Here's how the part is built. I have some questions about the finished solid (model axes, mm). A direction names the side the tool comes from. Coordinates: 2 decimals unless noted, no trailing zeros. Write each loop counter-clockwise with the first axis right and the second up, starting at its lowest first coordinate (ties: lowest second). Pieces come first, ordered by that corner, then holes. Notation, with made-up numbers: M -30,24.5 L -15,24.5 A12 cw -15,40.5 Z; hole C 81.5,87 d10. An arc over 180 degrees is marked long. Use a Markdown table: item, result.
```python
from build123d import *

# Parameters (mm, degrees)
ESQUISSE1_R             = 110
BOSS_EXTRU_1_DEPTH      = 50
BOSS_EXTRU_2_DEPTH      = 50
ESQUISSE3_R             = 20
ENL_V_MAT_EXTRU_1_DEPTH = 456.460206824
BOSS_EXTRU_3_DEPTH      = 30
BOSS_EXTRU_4_DEPTH      = 85


with BuildPart() as part:
    # Esquisse1 → Boss.-Extru.1 (new body)
    with BuildSketch(Plane(origin=(0, 0, 0), x_dir=(1, 0, 0), z_dir=(0, 1, 0))):
        with Locations(Location((0, 0, 0), (0, 0, 270))):
            Circle(ESQUISSE1_R)
    extrude(amount=BOSS_EXTRU_1_DEPTH)

    # Esquisse2 → Boss.-Extru.2 (add, symmetric)
    with BuildSketch(Plane.XY):
        with BuildLine():
            Line((-70, 45), (70, 45))
            Line((70, 45), (60, 352))
            ThreePointArc((60, 352), (0, 412), (-60, 352))
            Line((-60, 352), (-70, 45))
        make_face()
    extrude(amount=BOSS_EXTRU_2_DEPTH, both=True)

    # Esquisse3 → Enl_v. mat.-Extru.1 (cut, through all)
    with BuildSketch(Plane.XY.offset(50)):
        with Locations((0, 352)):
            Circle(ESQUISSE3_R)
    extrude(amount=-ENL_V_MAT_EXTRU_1_DEPTH, mode=Mode.SUBTRACT)

    # Esquisse4 → Boss.-Extru.3 (add)
    with BuildSketch(Plane(origin=(0, 0, -50), x_dir=(-1, 0, 0), z_dir=(0, 0, -1))):
        with BuildLine():
            Line((-38.056922747, 327.986032584), (56.171624225, 178.654251186))
            ThreePointArc((56.171624225, 178.654251186), (110.379680267, 165.580984438), (124.982074019, 219.397280669))
            Line((124.982074019, 219.397280669), (39.354833271, 373.821940753))
            ThreePointArc((39.354833271, 373.821940753), (-22.9271403, 390.721392507), (-38.056922747, 327.986032584))
        make_face()
    extrude(amount=BOSS_EXTRU_3_DEPTH)

    # Esquisse5 → Boss.-Extru.4 (add)
    with BuildSketch(Plane(origin=(0, 0, -80), x_dir=(-1, 0, 0), z_dir=(0, 0, -1))):
        with BuildLine():
            Line((56, 160), (124, 160))
            ThreePointArc((124, 160), (128.242640687, 161.757359313), (130, 166))
            Line((130, 166), (130, 234))
            ThreePointArc((130, 234), (128.242640687, 238.242640687), (124, 240))
            Line((124, 240), (56, 240))
            ThreePointArc((56, 240), (51.757359313, 238.242640687), (50, 234))
            Line((50, 234), (50, 166))
            ThreePointArc((50, 166), (51.757359313, 161.757359313), (56, 160))
        make_face()
    extrude(amount=BOSS_EXTRU_4_DEPTH)


solid = part.part
```
1. Will these pins go through, and if not, where does the flat tip stop? pin 1 Ø8 at (x, y) = (-16.5, 224) entering from -Z; pin 2 Ø12 at (x, y) = (-24.5, 293) entering from +Z; pin 3 Ø1.5 at (y, z) = (80.5, -9.5) entering from -X; pin 4 Ø6 at (y, z) = (94.5, -55) entering from +X.
Answers follow:
| item | result |
|---|---|
| pin 1 | stops at z = -50 |
| pin 2 | stops at z = 50 |
| pin 3 | stops at x = -68.87 |
| pin 4 | passes through |
2. Which directions (+Z, -Z, +X, -X, +Y, -Y) give clear straight access to the entire face, cutting with the end or side of a thin tool? Please do faces 4 (the face through (1.5, 50, -50.4)), 5 (the face through (-90, 240, -122)), 6 (the face through (-1, 234, 50)).
Answers follow:
| item | result |
|---|---|
| face 4 | none |
| face 5 | -Z, +X, -X, +Y |
| face 6 | +Z, +X, -X, +Y |
3. We'd pull the mould along Y, two halves only. Please class faces 1 (the face through (-50, 200, -122)), 2 (the face through (2, 0, -2)), 3 (the face through (15, 193, -50)): +Y half, -Y half, draft (parallel to the pull), parting line (faces both ways), or undercut.
Answers follow:
| item | result |
|---|---|
| face 1 | draft |
| face 2 | -Y half |
| face 3 | undercut |
4. Suppose I cut it at D-D on z = 84.5. Write out the boundary of the cut face in (x, y).
Answers follow:
| item | result |
|---|---|
| outline | M -70.43,0 L 70.43,0 L 70.43,50 L -70.43,50 Z |
5. Suppose I cut it at B-B on x = -11.5. Write out the boundary of the cut face in (y, z).
Answers follow:
| item | result |
|---|---|
| outline | M 0,-109.4 L 50,-109.4 L 50,-50 L 249.45,-50 L 249.45,-80 L 395.51,-80 L 395.51,-50 L 410.89,-50 L 410.89,50 L 368.36,50 L 368.36,-50 L 335.64,-50 L 335.64,50 L 50,50 L 50,109.4 L 0,109.4 Z |
6. I need wall thicknesses on probe 1 along Y at (x, z) = (0, 22); probe 2 along Y at (x, z) = (33, -82); probe 3 along Z at (x, y) = (-54, 83.5). Which ranges of each line are inside material? Lowest first, please.
Answers follow:
| item | result |
|---|---|
| probe 1 | y = 0 to 332, 372 to 412 |
| probe 2 | y = 0 to 50 |
| probe 3 | z = -50 to 50 |
7. Suppose I cut it at C-C on y = 205.5. Write out the boundary of the cut face in (x, z), and give its area (3 significant figures).
Answers follow:
| item | result |
|---|---|
| outline | M -130,-165 L -50,-165 L -50,-80 L -39.23,-80 L -39.23,-50 L 64.77,-50 L 64.77,50 L -64.77,50 L -64.77,-50 L -129.62,-50 L -129.62,-80 L -130,-80 Z |
| area | 22,500 mm2 |
8. Suppose I cut it at A-A on z = 0. Write out the boundary of the cut face in (x, y).
Answers follow:
| item | result |
|---|---|
| outline | M -110,0 L 110,0 L 110,50 L 69.84,50 L 60,352 A60 ccw -60,352 L -69.84,50 L -110,50 Z; hole C 0,352 d40 |
